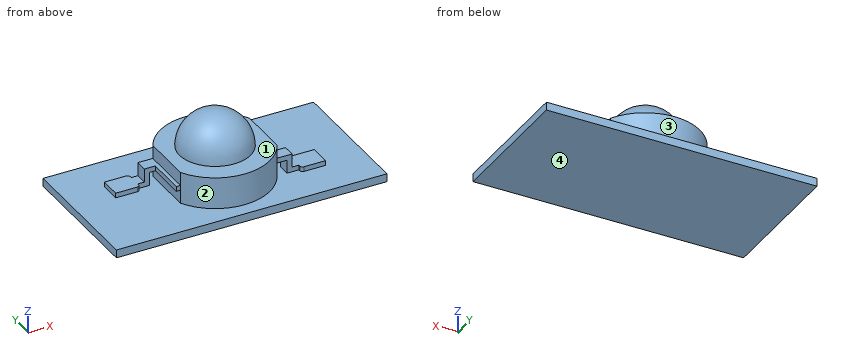
from build123d import *

# Parameters (mm, degrees)
SKETCH1_R            = 4.05
BOSS_EXTRUDE1_DEPTH  = 2.35
SKETCH2_R            = 1.5
SKETCH2_W            = 1
SKETCH2_H            = 1
BOSS_EXTRUDE2_DEPTH  = 0.2
REVOLVE1_ANGLE       = 180
SKETCH4_W            = 0.475
SKETCH4_H            = 8.1
CUT_EXTRUDE1_DEPTH   = 10.428845369
SKETCH5_W            = 0.37
SKETCH5_H            = 3.806244868
BOSS_EXTRUDE3_DEPTH  = 0.3
SKETCH6_W            = 0.37
SKETCH6_H            = 0.9
BOSS_EXTRUDE4_DEPTH  = 0.8
SKETCH7_W            = 0.37
SKETCH7_H            = 0.9
BOSS_EXTRUDE5_DEPTH  = 1
SKETCH8_W            = 0.5
SKETCH8_H            = 0.9
BOSS_EXTRUDE6_DEPTH  = 0.37
SKETCH9_W            = 0.37
SKETCH9_H            = 3.806244868
BOSS_EXTRUDE7_DEPTH  = 0.3
SKETCH10_W           = 0.37
SKETCH10_H           = 0.9
BOSS_EXTRUDE8_DEPTH  = 0.8
SKETCH11_W           = 0.37
SKETCH11_H           = 0.9
BOSS_EXTRUDE9_DEPTH  = 1
SKETCH12_W           = 0.5
SKETCH12_H           = 0.9
BOSS_EXTRUDE10_DEPTH = 0.37
SKETCH13_R           = 2.75
BOSS_EXTRUDE11_DEPTH = 0.1
SKETCH14_W           = 20
SKETCH14_H           = 10.1
BOSS_EXTRUDE13_DEPTH = 0.6


with BuildPart() as part:
    # Sketch1 → Boss-Extrude1 (new body)
    with BuildSketch(Plane.XY):
        with Locations((0, 4.05)):
            Circle(SKETCH1_R)
    extrude(amount=BOSS_EXTRUDE1_DEPTH)

    # Sketch2 → Boss-Extrude2 (add)
    with BuildSketch(Plane.XY.offset(2.35)):
        with Locations((0, 4.05)):
            Circle(SKETCH2_R)
        with Locations((0, 4.05)):
            Rectangle(SKETCH2_W, SKETCH2_H, mode=Mode.SUBTRACT)
    extrude(amount=BOSS_EXTRUDE2_DEPTH)

    # Sketch3 → Revolve1 (revolve)
    with BuildSketch(Plane.XY.offset(2.35)):
        with BuildLine():
            Line((-2.625, 4.05), (-2.5, 4.05))
            ThreePointArc((-2.5, 4.05), (0, 6.55), (2.5, 4.05))
            Line((2.5, 4.05), (2.625, 4.05))
            ThreePointArc((2.625, 4.05), (0, 6.675), (-2.625, 4.05))
        make_face()
    revolve(axis=Axis((0, 4.05, 2.35), (1, 0, 0)), revolution_arc=REVOLVE1_ANGLE)

    # Sketch4 → Cut-Extrude1 (cut, through all)
    with BuildSketch(Plane.XY.offset(2.35)):
        with Locations((-3.8125, 4.05)):
            Rectangle(SKETCH4_W, SKETCH4_H)
        with Locations((3.8125, 4.05)):
            Rectangle(SKETCH4_W, SKETCH4_H)
    extrude(amount=-CUT_EXTRUDE1_DEPTH, mode=Mode.SUBTRACT)

    # Sketch5 → Boss-Extrude3 (add)
    with BuildSketch(Plane.ZY.offset(3.575)):
        with Locations((1.175, 4.05)):
            Rectangle(SKETCH5_W, SKETCH5_H)
    extrude(amount=BOSS_EXTRUDE3_DEPTH)

    # Sketch6 → Boss-Extrude4 (add)
    with BuildSketch(Plane.ZY.offset(3.875)):
        with Locations((1.175, 5.503122434)):
            Rectangle(SKETCH6_W, SKETCH6_H)
    extrude(amount=BOSS_EXTRUDE4_DEPTH)

    # Sketch7 → Boss-Extrude5 (add)
    with BuildSketch(Plane(origin=(0, 0, 0.99), x_dir=(-1, 0, 0), z_dir=(0, 0, -1))):
        with Locations((4.49, 5.503122434)):
            Rectangle(SKETCH7_W, SKETCH7_H)
    extrude(amount=BOSS_EXTRUDE5_DEPTH)

    # Sketch8 → Boss-Extrude6 (add)
    with BuildSketch(Plane(origin=(0, 0, -0.01), x_dir=(-1, 0, 0), z_dir=(0, 0, -1))):
        with BuildLine():
            Line((5.175, 6.083122434), (5.175, 5.953122434))
            Line((5.175, 5.953122434), (5.175, 5.503122434))
            Line((5.175, 5.503122434), (6.975, 5.503122434))
            Line((6.975, 5.503122434), (6.975, 6.283122434))
            Line((6.975, 6.283122434), (5.375, 6.283122434))
            ThreePointArc((5.375, 6.283122434), (5.233578644, 6.224543791), (5.175, 6.083122434))
        make_face()
        with BuildLine():
            Line((6.975, 5.503122434), (5.175, 5.503122434))
            Line((5.175, 5.503122434), (5.175, 5.053122434))
            Line((5.175, 5.053122434), (5.175, 4.923122434))
            ThreePointArc((5.175, 4.923122434), (5.233578644, 4.781701078), (5.375, 4.723122434))
            Line((5.375, 4.723122434), (6.975, 4.723122434))
            Line((6.975, 4.723122434), (6.975, 5.503122434))
        make_face()
        with Locations((4.925, 5.503122434)):
            Rectangle(SKETCH8_W, SKETCH8_H)
    extrude(amount=-BOSS_EXTRUDE6_DEPTH)

    # Sketch9 → Boss-Extrude7 (add)
    with BuildSketch(Plane(origin=(3.575, 0, 0), x_dir=(0, 0, -1), z_dir=(1, 0, 0))):
        with Locations((-1.175, 4.05)):
            Rectangle(SKETCH9_W, SKETCH9_H)
    extrude(amount=BOSS_EXTRUDE7_DEPTH)

    # Sketch10 → Boss-Extrude8 (add)
    with BuildSketch(Plane(origin=(3.875, 0, 0), x_dir=(0, 0, -1), z_dir=(1, 0, 0))):
        with Locations((-1.175, 2.596877566)):
            Rectangle(SKETCH10_W, SKETCH10_H)
    extrude(amount=BOSS_EXTRUDE8_DEPTH)

    # Sketch11 → Boss-Extrude9 (add)
    with BuildSketch(Plane(origin=(0, 0, 0.99), x_dir=(-1, 0, 0), z_dir=(0, 0, -1))):
        with Locations((-4.49, 2.596877566)):
            Rectangle(SKETCH11_W, SKETCH11_H)
    extrude(amount=BOSS_EXTRUDE9_DEPTH)

    # Sketch12 → Boss-Extrude10 (add)
    with BuildSketch(Plane(origin=(0, 0, -0.01), x_dir=(-1, 0, 0), z_dir=(0, 0, -1))):
        with Locations((-4.925, 2.596877566)):
            Rectangle(SKETCH12_W, SKETCH12_H)
        with BuildLine():
            Line((-5.175, 2.016877566), (-5.175, 2.146877566))
            Line((-5.175, 2.146877566), (-5.175, 2.596877566))
            Line((-5.175, 2.596877566), (-6.975, 2.596877566))
            Line((-6.975, 2.596877566), (-6.975, 1.816877566))
            Line((-6.975, 1.816877566), (-5.375, 1.816877566))
            ThreePointArc((-5.375, 1.816877566), (-5.233578644, 1.875456209), (-5.175, 2.016877566))
        make_face()
        with BuildLine():
            Line((-6.975, 2.596877566), (-5.175, 2.596877566))
            Line((-5.175, 2.596877566), (-5.175, 3.046877566))
            Line((-5.175, 3.046877566), (-5.175, 3.176877566))
            ThreePointArc((-5.175, 3.176877566), (-5.233578644, 3.318298922), (-5.375, 3.376877566))
            Line((-5.375, 3.376877566), (-6.975, 3.376877566))
            Line((-6.975, 3.376877566), (-6.975, 2.596877566))
        make_face()
    extrude(amount=-BOSS_EXTRUDE10_DEPTH)

    # Sketch13 → Boss-Extrude11 (add)
    with BuildSketch(Plane(origin=(0, 0, 0), x_dir=(-1, 0, 0), z_dir=(0, 0, -1))):
        with Locations((0, 4.05)):
            Circle(SKETCH13_R)
    extrude(amount=BOSS_EXTRUDE11_DEPTH)

    # Sketch14 → Boss-Extrude13 (add)
    with BuildSketch(Plane(origin=(0, 0, 0), x_dir=(-1, 0, 0), z_dir=(0, 0, -1))):
        with Locations((0, 4.05)):
            Rectangle(SKETCH14_W, SKETCH14_H)
    extrude(amount=BOSS_EXTRUDE13_DEPTH)


solid = part.part
CAD build for the part. Positions are in the model's coordinates, mm. Face numbers are marked on the shaded views. A direction names the side the tool comes from. Coordinates: 2 decimals unless noted, no trailing zeros. Order: outer loops, then holes, each group sorted by start corner. A loop starts at its lowest first (then second) coordinate and runs counter-clockwise, first axis right, second up.
Item 1: Band-saw the part on D-D on y = 5.75. List the corners of the cut face in (x, z) (3 decimals), plus the area to 3 significant figures.
Check sheet entries:
outline: (-10, -0.6) - (10, -0.6) - (10, 0) - (3.575, 0) - (3.575, 0.99) - (3.875, 0.99) - (3.875, 1.36) - (3.575, 1.36) - (3.575, 2.35) - (2, 2.35) arc R2 ccw to (-2, 2.35) - (-3.575, 2.35) - (-3.575, 1.36) - (-4.675, 1.36) - (-4.675, 0.36) - (-6.975, 0.36) - (-6.975, 0) - (-10, 0) - close; hole (-4.305, 0) - (-3.575, 0) - (-3.575, 0.99) - (-4.305, 0.99) - close; hole (-1.833, 2.35) - (1.833, 2.35) arc R1.833 ccw to start
area: 31.5 mm2
Item 2: Band-saw the part on C-C on x = 5.75. List the corners of the cut face in (y, z).
Check sheet entries:
outline: (-1, -0.6) - (9.1, -0.6) - (9.1, 0) - (3.38, 0) - (3.38, 0.36) - (1.82, 0.36) - (1.82, 0) - (-1, 0) - close
Item 3: Band-saw the part on A-A on x = 0. List the corners of the cut face in (y, z) (3 decimals), plus the area to 3 significant figures.
Check sheet entries:
outline: (-1, -0.6) - (9.1, -0.6) - (9.1, 0) - (8.1, 0) - (8.1, 2.35) - (6.675, 2.35) arc R2.625 ccw to (1.425, 2.35) - (0, 2.35) - (0, 0) - (-1, 0) - close; hole (1.55, 2.35) - (2.55, 2.35) - (2.55, 2.55) - (3.55, 2.55) - (3.55, 2.35) - (4.55, 2.35) - (4.55, 2.55) - (5.55, 2.55) - (5.55, 2.35) - (6.55, 2.35) arc R2.5 ccw to start
area: 26.5 mm2
Item 4: 3-axis set-ups, long thin cutter, end or side, ignore diameter. For the marked faces 1, 2, 3 and 4: which of +Z, -Z, +X, -X, +Y, -Y reach the whole face in a straight line?
Check sheet entries:
face 1: +Z
face 2: +Z, -Y
face 3: +Z, +Y
face 4: -Z, +X, -X, +Y, -Y
Item 5: Drill centre lines: L1, parallel to X at y = 6, z = 3.25; L2, parallel to X at y = 3, z = 3.9; L3, parallel to Z at x = 3.25, y = 7.75. Where is each one in solid material? Low to high.
Check sheet entries:
L1: x = -1.51 to -1.28, 1.28 to 1.51
L2: x = -1.84 to -1.66, 1.66 to 1.84
L3: z = -0.6 to 0
Item 6: Pin check, flat tips, straight feed: pin 1 Ø1.5 at (x, z) = (-1, 1) entering from -Y; pin 2 Ø1.5 at (x, y) = (-1, 4.5) entering from +Z; pin 3 Ø1 at (x, y) = (-7.5, 1.5) entering from +Z. Stop position of each tip, or through.
Check sheet entries:
pin 1: stops at y = 0.01
pin 2: stops at z = 4.95
pin 3: stops at z = 0
Item 7: Band-saw the part on B-B on y = 4.05. List the corners of the cut face in (x, z) (3 decimals), plus the area to 3 significant figures.
Check sheet entries:
outline: (-10, -0.6) - (10, -0.6) - (10, 0) - (3.575, 0) - (3.575, 0.99) - (3.875, 0.99) - (3.875, 1.36) - (3.575, 1.36) - (3.575, 2.35) - (2.625, 2.35) arc R2.625 ccw to (-2.625, 2.35) - (-3.575, 2.35) - (-3.575, 1.36) - (-3.875, 1.36) - (-3.875, 0.99) - (-3.575, 0.99) - (-3.575, 0) - (-10, 0) - close; hole (-2.5, 2.35) - (-1.5, 2.35) - (-1.5, 2.55) - (-0.5, 2.55) - (-0.5, 2.35) - (0.5, 2.35) - (0.5, 2.55) - (1.5, 2.55) - (1.5, 2.35) - (2.5, 2.35) arc R2.5 ccw to start
area: 30.4 mm2
